Work out the finished part from the listing and answer in its coordinate system (mm). Face numbers are marked on the shaded views. A direction names the side the tool comes from. Round coordinates to 2 decimals unless told otherwise and drop trailing zeros. Order: outer loops, then holes, each group sorted by start corner. A loop starts at its lowest first (then second) coordinate and runs counter-clockwise, first axis right, second up. Notation, with made-up numbers: (-36, 3) - (14, 3) arc R9 cw to (14, 17) - close; hole circle Ø9 at (35, -23.5). An arc over 180 degrees is marked (long way). Use one line per item in the form item = value. Start each with the question number.
Q1. For a pull along Y with two mould halves and no side action, classify the marked faces 1, 2 and 3 as +Y half, -Y half, draft (parallel to the pull), parting line (faces both ways), or undercut.
Q2. Given P1, Ø1, axis at y = -511.5, z = 198, coming from the -X side; P2, Ø1.5, axis at x = 2, z = 37, coming from the -Y side; P3, Ø12, axis at y = -515.5, z = 55.5, coming from the +X side; P4, Ø4, axis at x = 370.5, y = 28, coming from the -Z side, each flat-ended and moving along its own axis, determine where each tip first touches the part or whether it passes through.
Q3. The part is cut by section A-A on x = 27. Determine the outline of the cut face in (y, z), plus the area to 3 significant figures.
Q4. Find the intervals of material crossed by line 1 (X direction, y = -76, z = 29); line 2 (X direction, y = -190.5, z = 282); line 3 (Y direction, x = -622.3, z = 29), in increasing order. Write a range as [from, to].
Q5. Which of the six approach directions +Z, -Z, +X, -X, +Y, -Y give full straight-line access (tool end or side, diameter ignored) to the marked faces 4, 5 and 6?
Q6. The part is cut by section B-B on y = -36. Determine the outline of the cut face in (x, z).
from build123d import *

# Parameters (mm, degrees)
F0_W      = 1358.9
F0_H      = 304.8
F0_R      = 20.6375
F1_DEPTH  = 50.8
F2_W      = 25.4
F2_H      = 304.8
F3_DEPTH  = 228.6
F5_DEPTH  = 1244.601
F6_W      = 203.2
F6_H      = 457.2
F7_DEPTH  = 298.45
F8_R      = 141.2875
F9_DEPTH  = 152.4
F10_R     = 111.125
F11_DEPTH = 1193.801
F13_D     = 19.84248
F13_DEPTH = 38.1
F13_TIP   = 5.9612824079
F15_D     = 19.84248
F15_DEPTH = 38.1
F15_TIP   = 5.9612824079
F18_DEPTH = 927.1


with BuildPart() as f1:
    # F0 (on Top) → F1 (new body)
    with BuildSketch(Plane.XY):
        Rectangle(F0_W, F0_H)
        with Locations((-622.3, -76.2)):
            Circle(F0_R, mode=Mode.SUBTRACT)
        with Locations((-482.6, -76.2)):
            Circle(F0_R, mode=Mode.SUBTRACT)
        with Locations((482.6, -76.2)):
            Circle(F0_R, mode=Mode.SUBTRACT)
        with Locations((622.3, -76.2)):
            Circle(F0_R, mode=Mode.SUBTRACT)
        with Locations((-622.3, 76.2)):
            Circle(F0_R, mode=Mode.SUBTRACT)
        with Locations((-482.6, 76.2)):
            Circle(F0_R, mode=Mode.SUBTRACT)
        with Locations((482.6, 76.2)):
            Circle(F0_R, mode=Mode.SUBTRACT)
        with Locations((622.3, 76.2)):
            Circle(F0_R, mode=Mode.SUBTRACT)
    extrude(amount=F1_DEPTH)

    # F2 (on face) → F3 (join)
    with BuildSketch(Plane.XY.offset(50.8)):
        with Locations((-552.45, 0)):
            Rectangle(F2_W, F2_H)
        with Locations((552.45, 0)):
            Rectangle(F2_W, F2_H)
    extrude(amount=F3_DEPTH)

    # F4 (on face) → F5 (cut, through all)
    with BuildSketch(Plane.YZ.offset(565.15)):
        Polygon((152.4, 279.4), (-101.6, 279.4), (152.4, 101.6), align=None)
    extrude(amount=-F5_DEPTH, mode=Mode.SUBTRACT)

    # F16: F7 across plane


with BuildPart() as f7:
    # F6 (on face) → F7 (new body)
    with BuildSketch(Plane(origin=(0, 0, 0), x_dir=(1, 0, 0), z_dir=(0, 0, -1))):
        with Locations((565.15, 381)):
            Rectangle(F6_W, F6_H)
    extrude(amount=-F7_DEPTH)

    # F8 (on face) → F9 (cut)
    with BuildSketch(Plane.YZ.offset(666.75)):
        with Locations((-381, 298.45)):
            Circle(F8_R)
    extrude(amount=-F9_DEPTH, mode=Mode.SUBTRACT)

    # F10 (on face) → F11 (cut, through all)
    with BuildSketch(Plane.YZ.offset(514.35)):
        with Locations((-381, 298.45)):
            Circle(F10_R)
    extrude(amount=-F11_DEPTH, mode=Mode.SUBTRACT)

    # F13
    with Locations(Plane.YZ.offset(666.75)):
        with Locations((-534.9793167929, 209.55), (-381, 120.65), (-227.0206832071, 209.55)):
            Hole(F13_D / 2, depth=F13_DEPTH)
            with Locations((0, 0, -(F13_DEPTH + F13_TIP / 2))):  # 118° drill point
                Cone(0, F13_D / 2, F13_TIP, mode=Mode.SUBTRACT)

    # F15
    with Locations(Plane.XY.offset(298.45)):
        with Locations((514.35, -571.5), (628.65, -571.5), (514.35, -190.5), (628.65, -190.5)):
            Hole(F15_D / 2, depth=F15_DEPTH)
            with Locations((0, 0, -(F15_DEPTH + F15_TIP / 2))):  # 118° drill point
                Cone(0, F15_D / 2, F15_TIP, mode=Mode.SUBTRACT)


with BuildPart() as f1_1:
    add(f1.part)
    add(f7.part.mirror(Plane.YZ))


    add(f7.part)  # F18 merges F7
    # F17 (on face) → F18 (join, through all)
    with BuildSketch(Plane.YZ.offset(-463.55)):
        Polygon((-596.9, 12.7), (-495.3, 12.7), (-495.3, 31.75), (-577.85, 31.75), (-577.85, 114.3), (-596.9, 114.3), align=None)
    extrude(amount=F18_DEPTH)


solid = f1_1.part
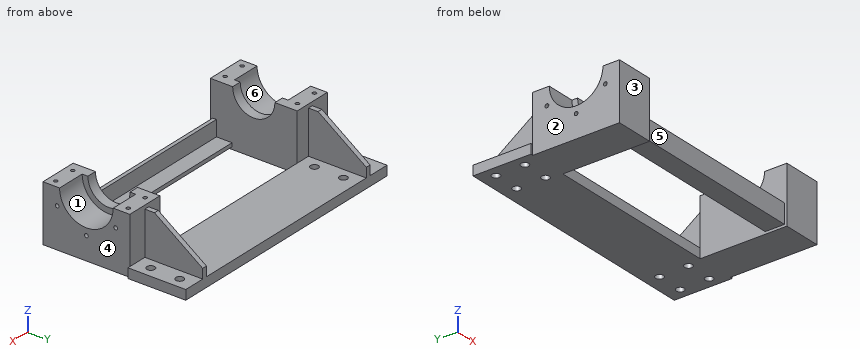
Found:
q1.face_1 = undercut
q1.face_2 = draft
q1.face_3 = -Y half
q2.P1 = -666.75
q2.P2 = -596.9
q2.P3 = 666.75
q2.P4 = 0
q3.outline = (-596.9, 12.7) - (-495.3, 12.7) - (-495.3, 31.75) - (-577.85, 31.75) - (-577.85, 114.3) - (-596.9, 114.3) - close; (-152.4, 0) - (152.4, 0) - (152.4, 50.8) - (-152.4, 50.8) - close
q3.area = 19,000 mm²
q4.line_1 = [-679.45, -642.94], [-601.66, -503.24], [-461.96, 461.96], [503.24, 601.66], [642.94, 679.45]
q4.line_2 = [-666.75, -638.57], [-618.73, -524.27], [-504.43, -463.55], [463.55, 504.43], [524.27, 618.73], [638.57, 666.75]
q4.line_3 = [-609.6, -96.84], [-55.56, 55.56], [96.84, 152.4]
q5.face_4 = +Z, -Z, +X, -Y
q5.face_5 = +Z, -Z, -Y
q5.face_6 = +Z, -X
q6.outline = (-679.45, 0) - (679.45, 0) - (679.45, 50.8) - (565.15, 50.8) - (565.15, 233.48) - (539.75, 233.48) - (539.75, 50.8) - (-539.75, 50.8) - (-539.75, 233.48) - (-565.15, 233.48) - (-565.15, 50.8) - (-679.45, 50.8) - close
